Design review of the part shown in the three views and the two pictorial views. Dimensions are in mm from the part's minimum x, y and z. A direction names the side the tool comes from. Coordinates: 2 decimals unless noted, no trailing zeros. Loops run counter-clockwise (first coordinate to the right, second up) from the corner with the lowest first, then second, coordinate; pieces in that order, holes last. Notation, with made-up numbers: M 81.5,32.25 L 134.5,32.25 A19 cw 134.5,63.25 Z; hole C 56,-4.75 d2. An arc over 180 degrees is marked long. Put each result on its own line as item: value. Start each with the question number.
(1) The part is to be moulded in two halves that separate along Z. For the marked faces 1, 2 and 3, say which applies: +Z half, -Z half, draft (parallel to the pull), parting line (faces both ways), or undercut.
(2) For the marked faces 4 and 5, list the 3-axis set-ups (+Z, -Z, +X, -X, +Y, -Y) from which the entire face can be reached by the end or side of a thin tool; tool diameter is ignored.
(3) Take a section at B-B, the plane y = 5. Give the boundary of the cut face in (x, z), then the cut area to 3 significant figures.
(4) Take a section at A-A, the plane z = 50. Give the boundary of the cut face in (x, y).
(5) Clearance check with flat-ended pins moving along their axes: pin 1 (3.5 mm diameter, centred on x = 91.5, z = 88.5, fed in from +Y); pin 2 (1.5 mm diameter, centred on x = 79, z = 65, fed in from -Y); pin 3 (6 mm diameter, centred on x = 10, z = 90, fed in from -Y). State where each tip first meets the part, or that it passes through.
(6) Take a section at C-C, the plane x = 10. Give the boundary of the cut face in (y, z).
(7) Take a section at D-D, the plane z = 10. Give the boundary of the cut face in (x, y).
(8) For probe 1 along Z at (x, y) = (90, 10.7); probe 2 along X at (y, z) = (2.5, 50); probe 3 along Z at (x, y) = (88, 5.5), list the stretches that pass through material, from the lowest coordinate up. Write a range as [from, to].
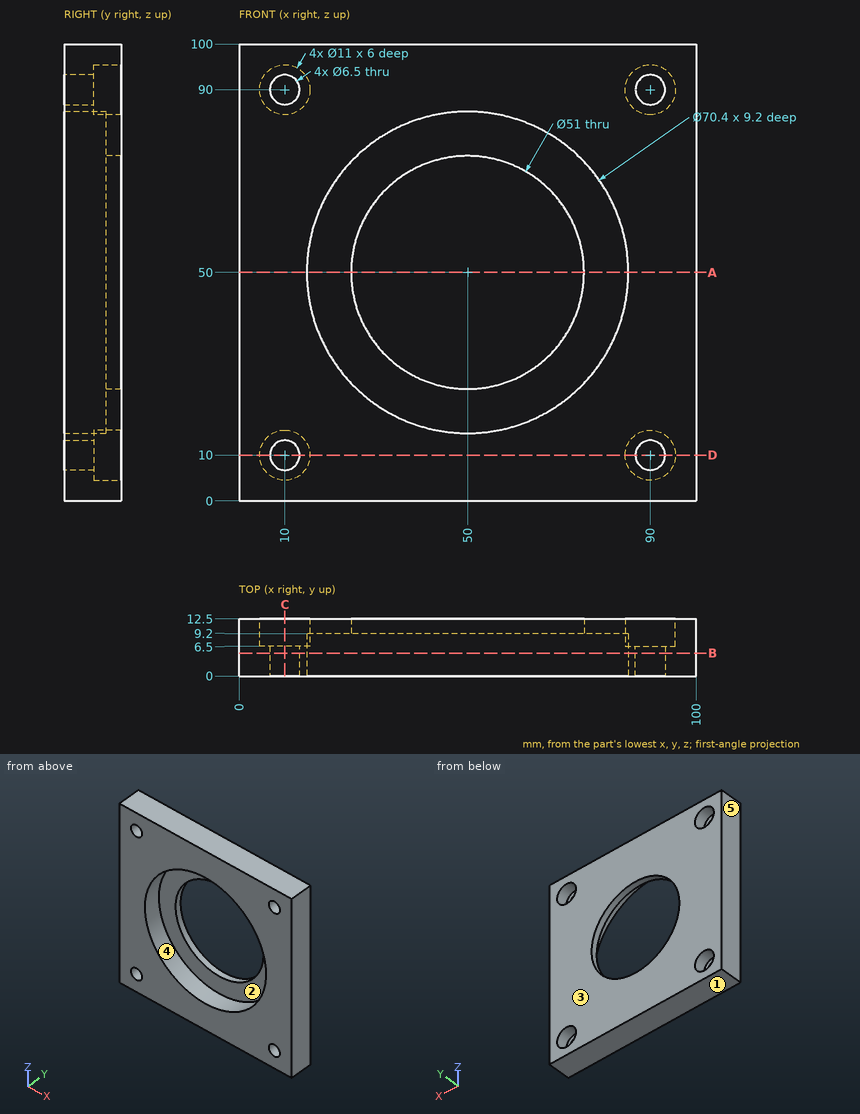
Computed values:
1. face 1: -Z half
1. face 2: undercut
1. face 3: draft
2. face 4: -Y
2. face 5: +Z, -Z, -X, +Y, -Y
3. outline: M 0,0 L 100,0 L 100,100 L 0,100 Z; hole C 10,10 d6.5; hole C 10,90 d6.5; hole C 50,50 d70.4; hole C 90,10 d6.5; hole C 90,90 d6.5
3. area: 5,970 mm^2
4. outline: M 0,0 L 14.8,0 L 14.8,9.2 L 24.5,9.2 L 24.5,12.5 L 0,12.5 Z; M 75.5,9.2 L 85.2,9.2 L 85.2,0 L 100,0 L 100,12.5 L 75.5,12.5 Z
5. pin 1: stops at y = 6.5
5. pin 2: stops at y = 9.2
5. pin 3: passes through
6. outline: M 0,0 L 12.5,0 L 12.5,4.5 L 6.5,4.5 L 6.5,6.75 L 0,6.75 Z; M 0,13.25 L 6.5,13.25 L 6.5,15.5 L 12.5,15.5 L 12.5,84.5 L 6.5,84.5 L 6.5,86.75 L 0,86.75 Z; M 0,93.25 L 6.5,93.25 L 6.5,95.5 L 12.5,95.5 L 12.5,100 L 0,100 Z
7. outline: M 0,0 L 6.75,0 L 6.75,6.5 L 4.5,6.5 L 4.5,12.5 L 0,12.5 Z; M 13.25,0 L 86.75,0 L 86.75,6.5 L 84.5,6.5 L 84.5,12.5 L 15.5,12.5 L 15.5,6.5 L 13.25,6.5 Z; M 93.25,0 L 100,0 L 100,12.5 L 95.5,12.5 L 95.5,6.5 L 93.25,6.5 Z
8. probe 1: z = [0, 4.5], [15.5, 84.5], [95.5, 100]
8. probe 2: x = [0, 14.8], [85.2, 100]
8. probe 3: z = [0, 7.44], [12.56, 87.44], [92.56, 100]
